```python
from build123d import *

# Parameters (mm, degrees)
F0_W     = 9
F0_H     = 9
F0_R     = 1.25
F1_DEPTH = 7
F2_DEPTH = 13


with BuildPart() as f1:
    # F0 (on Top) → F1 (new body)
    with BuildSketch(Plane.XY):
        with Locations((-42.070914, 24.336671)):
            Rectangle(F0_W, F0_H)
        with Locations((-42.070914, 24.336671)):
            Circle(F0_R, mode=Mode.SUBTRACT)
        Polygon((-49.570914, 16.836671), (-37.570914, 16.836671), (-37.570914, 19.836671), (-46.570914, 19.836671), (-46.570914, 28.836671), (-49.570914, 28.836671), align=None)
    extrude(amount=F1_DEPTH)

    # F0 (on Top) → F2 (join)
    with BuildSketch(Plane.XY):
        Polygon((-49.570914, 16.836671), (-37.570914, 16.836671), (-37.570914, 19.836671), (-46.570914, 19.836671), (-46.570914, 28.836671), (-49.570914, 28.836671), align=None)
    extrude(amount=F2_DEPTH)


solid = f1.part
```
Can you work these out from the model? Positions are in its coordinate system, mm. A direction names the side the tool comes from. Round coordinates to 2 decimals unless told otherwise and drop trailing zeros. Loops run counter-clockwise (first coordinate to the right, second up) from the corner with the lowest first, then second, coordinate; pieces in that order, holes last. Notation, with made-up numbers: (42, 1.5) -> (59, 1.5) arc R24 ccw to (59, 37.5) -> close; hole circle Ø1 at (78.5, 79). An arc over 180 degrees is marked (long way). One line per item, written item: value. Start each with the question number.
1. For faces 1 (the flat face through (-43, 23, 7)), 2 (the flat face through (-37.571, 21, 5)), which set-ups out of +Z, -Z, +X, -X, +Y, -Y let a thin tool reach every point of the face, with its end or its side?
2. If I drill on probe 1 along Z at (x, y) = (-43.5, 23.5); probe 2 along Y at (x, z) = (-45.25, 9.5); probe 3 along X at (y, z) = (21, 11.5), over which ranges is the centre line in solid material (lowest first)?
3. If we section it at B-B, the plane z = 9.25: Write out the boundary of the cut face in (x, y), then the cut area to 3 significant figures.
4. If we mould it in two halves opening along X, with no side actions, what happens to faces 3 (the cylindrical face through (-41.4, 25.39, 3.45)), 4 (the flat face through (-46, 19, 13)), 5 (the flat face through (-46.571, 24, 10))? For each: pulls with the +X half, pulls with the -X half, needs draft (parallel to the pull), parting line crosses it, or undercut.
5. For pin 1 (1.8 mm diameter, centred on y = 24.5, z = 11, fed in from +X); pin 2 (1.8 mm diameter, centred on x = -42.5, z = 9, fed in from +Y), each with a flat end and sliding along its axis, tell me the tip position at first contact or that it passes through.
6. If we section it at C-C, the plane y = 23.5: Write out the boundary of the cut face in (x, z).
7. If we section it at A-A, the plane x = -41: Write out the boundary of the cut face in (y, z), then the cut area to 3 significant figures.
8. If we section it at D-D, the plane y = 20.5: Write out the boundary of the cut face in (x, z).
Calculated:
1. face 1: +Z, +X, +Y
1. face 2: +Z, -Z, +X, +Y, -Y
2. probe 1: z = 0 to 7
2. probe 2: y = 16.84 to 19.84
2. probe 3: x = -49.57 to -46.57
3. outline: (-49.57, 16.84) -> (-37.57, 16.84) -> (-37.57, 19.84) -> (-46.57, 19.84) -> (-46.57, 28.84) -> (-49.57, 28.84) -> close
3. area: 63.0 mm²
4. face 3: undercut
4. face 4: needs draft
4. face 5: pulls with the +X half
5. pin 1: stops at x = -46.57
5. pin 2: stops at y = 19.84
6. outline: (-49.57, 0) -> (-43, 0) -> (-43, 7) -> (-46.57, 7) -> (-46.57, 13) -> (-49.57, 13) -> close; (-41.14, 0) -> (-37.57, 0) -> (-37.57, 7) -> (-41.14, 7) -> close
7. outline: (16.84, 0) -> (23.69, 0) -> (23.69, 7) -> (19.84, 7) -> (19.84, 13) -> (16.84, 13) -> close; (24.98, 0) -> (28.84, 0) -> (28.84, 7) -> (24.98, 7) -> close
7. area: 93.0 mm²
8. outline: (-49.57, 0) -> (-37.57, 0) -> (-37.57, 7) -> (-46.57, 7) -> (-46.57, 13) -> (-49.57, 13) -> close
